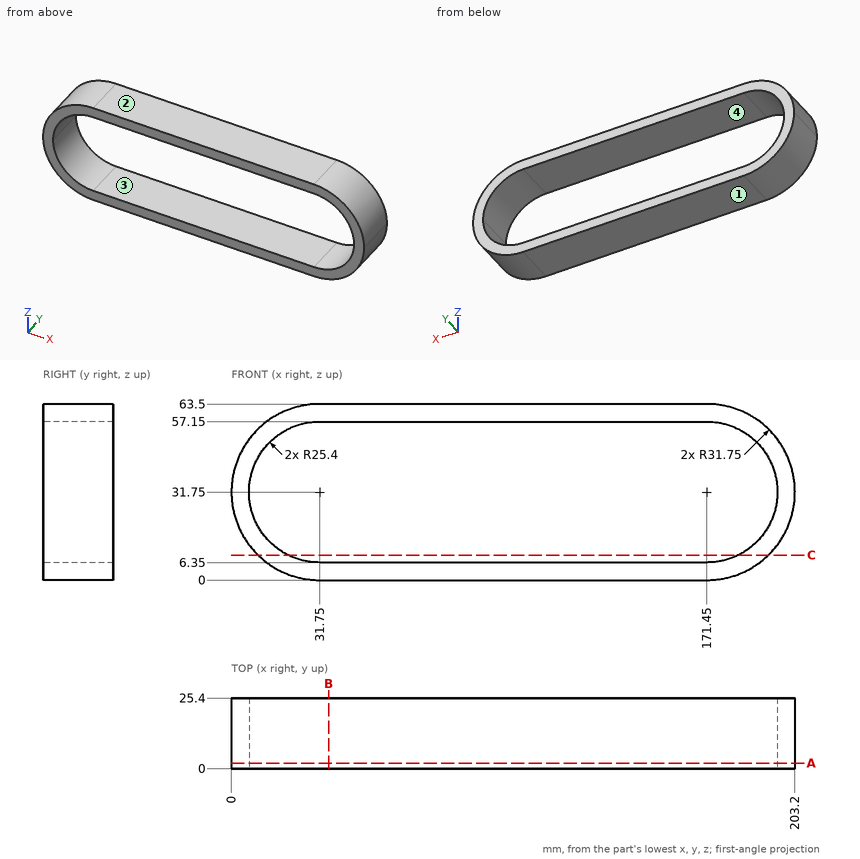
Study the drawing (mm; zero at the part's minimum x, y, z) and answer. Coordinates: 2 decimals unless noted, no trailing zeros. Loops run counter-clockwise (first coordinate to the right, second up) from the corner with the lowest first, then second, coordinate; pieces in that order, holes last. Notation, with made-up numbers: M 83,7 L 113,7 A35 ccw 113,44 Z; hole C 52,33.25 d8. An arc over 180 degrees is marked long. Answer as a JSON object with one key per item and string values. Group by question number.
Item 1: Section C-C (z = 9) is taken. Write down the section's boundary in (x, y), and give its area (3 significant figures).
Item 2: Determine the mould class of the marked faces 1, 2, 3 and 4 for opening direction Z: +Z half, -Z half, draft (parallel to the pull), parting line (faces both ways), or undercut.
Item 3: Section B-B (x = 35) is taken. Write down the section's boundary in (y, z).
Item 4: Section A-A (y = 2) is taken. Write down the section's boundary in (x, z), and give its area (3 significant figures).
Item 5: Each of these flat-tipped pins is pushed along its axis until it touches: P1, Ø4, axis at x = 175, y = 10, coming from the -Z side; P2, Ø1.5, axis at y = 11.5, z = 26, coming from the -X side; P3, Ø10, axis at y = 19.5, z = 44.5, coming from the -X side. Where does it stop, or does it pass through?
Item 6: Consider L1, parallel to Z at x = 53, y = 7.25; L2, parallel to X at y = 5.25, z = 31; L3, parallel to X at y = 9.75, z = 17.5. Determine where each line is inside the solid, lowest interval first.
Solved:
{
 "1": {"outline": "M 9.6,0 L 20.45,0 L 20.45,25.4 L 9.6,25.4 Z; M 182.75,0 L 193.6,0 L 193.6,25.4 L 182.75,25.4 Z", "area": "551 mm2"},
 "2": {"face 1": "-Z half", "face 2": "+Z half", "face 3": "undercut", "face 4": "undercut"},
 "3": {"outline": "M 0,0 L 25.4,0 L 25.4,6.35 L 0,6.35 Z; M 0,57.15 L 25.4,57.15 L 25.4,63.5 L 0,63.5 Z"},
 "4": {"outline": "M 0,31.75 A31.75 ccw 31.75,0 L 171.45,0 A31.75 ccw 203.2,31.75 A31.75 ccw 171.45,63.5 L 31.75,63.5 A31.75 ccw Z; hole M 6.35,31.75 A25.4 ccw 31.75,6.35 L 171.45,6.35 A25.4 ccw 196.85,31.75 A25.4 ccw 171.45,57.15 L 31.75,57.15 A25.4 ccw Z", "area": "2,910 mm2"},
 "5": {"P1": "stops at z = 0.04", "P2": "stops at x = 0.4", "P3": "stops at x = 0.96"},
 "6": {"L1": "z = 0 to 6.35, 57.15 to 63.5", "L2": "x = 0.01 to 6.36, 196.84 to 203.19", "L3": "x = 3.38 to 10.72, 192.48 to 199.82"}
}
